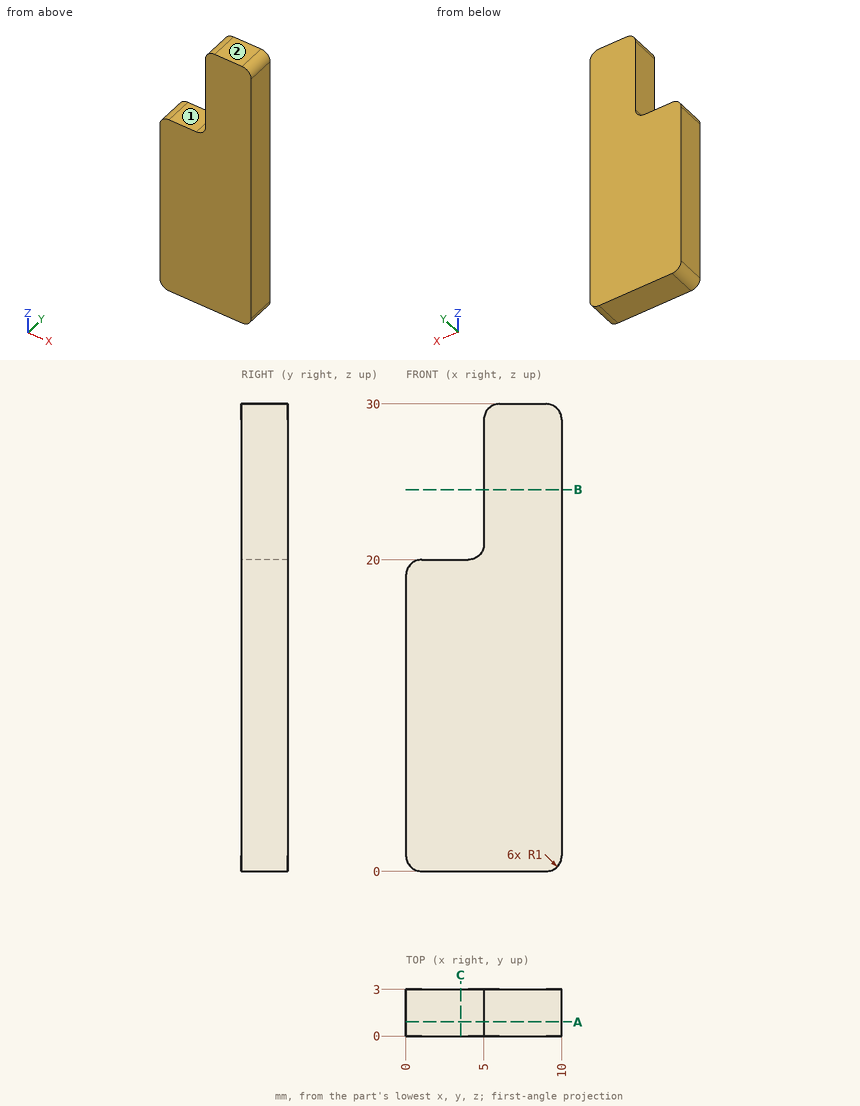
Geometry: see drawing. Coordinates: mm, zero at the bounding-box minimum. A direction names the side the tool comes from. Round coordinates to 2 decimals unless told otherwise and drop trailing zeros. Order: outer loops, then holes, each group sorted by start corner. A loop starts at its lowest first (then second) coordinate and runs counter-clockwise, first axis right, second up. Notation, with made-up numbers: (-37, -14.75) - (-2, -14.75) arc R27 ccw to (-2, 18.25) - close; hole circle Ø5 at (83.5, 5.25). An arc over 180 degrees is marked (long way). Use a Markdown table: item, result. Add a question column.
1. Section query A-A (y = 0.9). Return the cut outline in (x, z).
2. Line query: probe 1 along X at (y, z) = (1.1, 24.75); probe 2 along Z at (x, y) = (2.75, 1.8); probe 3 along Z at (x, y) = (4.75, 1.55). Output: solid intervals per line, ascending.
3. Section query C-C (x = 3.5). Return the cut outline in (y, z), then the cut area to 3 significant figures.
4. Set-up query: the marked faces 1 and 2. Return all of +Z, -Z, +X, -X, +Y, -Y with unobstructed straight access to the full face (end or side cutting, diameter ignored); none if empty.
5. First-contact query: pin 1 (1.5 mm diameter, centred on x = 3, y = 1, fed in from +Z); pin 2 (1.5 mm diameter, centred on y = 2, z = 27, fed in from -X). Flat tips, straight axial feed; report the tip coordinate or a pass-through.
6. Section query B-B (z = 24.5). Return the cut outline in (x, y).
Derived:
| question | item | result |
|---|---|---|
| 1 | outline | (0, 1) arc R1 ccw to (1, 0) - (9, 0) arc R1 ccw to (10, 1) - (10, 29) arc R1 ccw to (9, 30) - (6, 30) arc R1 ccw to (5, 29) - (5, 21) arc R1 cw to (4, 20) - (1, 20) arc R1 ccw to (0, 19) - close |
| 2 | probe 1 | 5 to 10 |
| 2 | probe 2 | 0 to 20 |
| 2 | probe 3 | 0 to 20.34 |
| 3 | outline | (0, 0) - (3, 0) - (3, 20) - (0, 20) - close |
| 3 | area | 60.0 mm2 |
| 4 | face 1 | +Z, -X, +Y, -Y |
| 4 | face 2 | +Z, +X, -X, +Y, -Y |
| 5 | pin 1 | z = 20 |
| 5 | pin 2 | x = 5 |
| 6 | outline | (5, 0) - (10, 0) - (10, 3) - (5, 3) - close |
